Check sheet for the modelled part. Datum: model origin and axes. Units: mm. A direction names the side the tool comes from. Round coordinates to 2 decimals unless told otherwise and drop trailing zeros. Order: outer loops, then holes, each group sorted by start corner. A loop starts at its lowest first (then second) coordinate and runs counter-clockwise, first axis right, second up.
```python
from build123d import *

# Parameters (mm, degrees)
F0_R     = 40
F0_R_2   = 34.9999991059
F5_R     = 75
F5_R_2   = 40
F6_DEPTH = 5
F2_R     = 4
F7_DEPTH = 5


with BuildPart() as f3:
    # F3: sweep along a path in F1
    with BuildLine(Plane.XZ) as f3_path:
        Line((0, 0), (100, 0))
        Line((100, 0), (100, 200))
    # F0 (on Right) → F3 (sweep)
    with BuildSketch(Plane.YZ):
        Circle(F0_R)
        Circle(F0_R_2, mode=Mode.SUBTRACT)
    sweep(path=f3_path.line, transition=Transition.RIGHT)

    # F5 (on face) → F6 (join)
    with BuildSketch(Plane.XY.offset(100)):
        with Locations((100, 0)):
            Circle(F5_R)
        with Locations((100, 0)):
            Circle(F5_R_2, mode=Mode.SUBTRACT)
    extrude(amount=-F6_DEPTH)

    # F2 (on Right) → F7 (join)
    with BuildSketch(Plane.YZ):
        with BuildLine():
            Line((-70, -75), (70, -75))
            ThreePointArc((70, -75), (73.5355339059, -73.5355339059), (75, -70))
            Line((75, -70), (75, 70))
            ThreePointArc((75, 70), (73.5355339059, 73.5355339059), (70, 75))
            Line((70, 75), (-70, 75))
            ThreePointArc((-70, 75), (-73.5355339059, 73.5355339059), (-75, 70))
            Line((-75, 70), (-75, -70))
            ThreePointArc((-75, -70), (-73.5355339059, -73.5355339059), (-70, -75))
        make_face()
        with Locations((-50, -45)):
            Circle(F2_R, mode=Mode.SUBTRACT)
        with Locations((50, -45)):
            Circle(F2_R, mode=Mode.SUBTRACT)
        with Locations((-50, 55)):
            Circle(F2_R, mode=Mode.SUBTRACT)
        with Locations((50, 55)):
            Circle(F2_R, mode=Mode.SUBTRACT)
    extrude(amount=F7_DEPTH)


solid = f3.part
```
Item 1: Access from +Z, -Z, +X, -X, +Y, -Y to the whole of each face (thin tool, end or side, straight path). Record for faces 5 (the cylindrical face through (134.168, -7.587, 110.256)), 6 (the cylindrical face through (56.466, -7.587, -34.168)), 7 (the cylindrical face through (2.46, 47.05, -42.3)).
Answer:
face 5: +Z
face 6: none
face 7: +X, -X
Item 2: Sectioned sample at D-D (y = -50). Record the cut outline in (x, z).
Answer:
outline: (0, -75) - (5, -75) - (5, -49) - (0, -49) - close; (0, -41) - (5, -41) - (5, 51) - (0, 51) - close; (0, 59) - (5, 59) - (5, 75) - (0, 75) - close; (44.1, 95) - (155.9, 95) - (155.9, 100) - (44.1, 100) - close
Item 3: Go/stop test with flat-tipped pins: P1, Ø12, axis at x = 137.5, z = 66, coming from the +Y side; P2, Ø1.5, axis at x = 3.5, y = 11, coming from the +Z side; P3, Ø9, axis at y = -50, z = 55, coming from the -X side; P4, Ø10, axis at x = 103, z = 138, coming from the -Y side. Record where each tip stops, or that it passes through.
Answer:
P1: stops at y = 24.65
P2: stops at z = 75
P3: stops at x = 0
P4: stops at y = -40
Item 4: Sectioned sample at B-B (z = 55). Record the cut outline in (x, y), and give its area (3 significant figures).
Answer:
outline: (0, -75) - (5, -75) - (5, -54) - (0, -54) - close; (0, -46) - (5, -46) - (5, 46) - (0, 46) - close; (0, 54) - (5, 54) - (5, 75) - (0, 75) - close; circle Ø80 at (100, 0); hole circle Ø70 at (100, 0)
area: 1,850 mm2
Item 5: Scan lines: line 1 along Z through (x, y) = (3.6, 50); line 2 along Z through (x, y) = (15, 1); line 3 along Z through (x, y) = (39, -16). Record each from-to range of solid material in increasing order.
Answer:
line 1: z = -75 to -49, -41 to 51, 59 to 75
line 2: z = -39.99 to -34.99, 34.99 to 39.99
line 3: z = -36.66 to -31.13, 31.13 to 36.66, 95 to 100
Item 6: Sectioned sample at C-C (x = 50). Record the cut outline in (y, z).
Answer:
outline: (-55.9, 95) - (55.9, 95) - (55.9, 100) - (-55.9, 100) - close; circle Ø80 at (0, 0); hole circle Ø70 at (0, 0)
Item 7: Sectioned sample at A-A (z = -45). Record the cut outline in (x, y).
Answer:
outline: (0, -75) - (5, -75) - (5, -54) - (0, -54) - close; (0, -46) - (5, -46) - (5, 46) - (0, 46) - close; (0, 54) - (5, 54) - (5, 75) - (0, 75) - close
Item 8: Release check for a two-part mould opening along Z. For faces 1 (the flat face through (99.8, -35.4, 200)), 2 (the cylindrical face through (2.465, 49.133, 51.095)), 3 (the cylindrical face through (87.985, 38.153, 150.7)), 4 (the flat face through (5, 0, 0)) record: released by +Z, released by -Z, zero draft, split by the parting line, or undercut.
Answer:
face 1: released by +Z
face 2: undercut
face 3: zero draft
face 4: undercut
